from build123d import *

# Parameters (mm, degrees)
SCHIZZO1_R                   = 7
SCHIZZO1_R_2                 = 1.5
ESTRUSIONE_ESTRUSIONE1_DEPTH = 3
ESTRUSIONE_ESTRUSIONE2_DEPTH = 22
SCHIZZO3_W                   = 10
SCHIZZO3_H                   = 3
SCHIZZO3_W_2                 = 3
SCHIZZO3_H_2                 = 21.5
ESTRUSIONE_ESTRUSIONE3_DEPTH = 5


with BuildPart() as part:
    # Schizzo1 → Estrusione-Estrusione1 (new body)
    with BuildSketch(Plane.XY):
        with BuildLine():
            Line((-132.593868151, -125.596865141), (-162.593868151, -125.596865141))
            Line((-162.593868151, -125.596865141), (-162.593868151, -112.596865141))
            ThreePointArc((-162.593868151, -112.596865141), (-162.055269261, -110.529315323), (-160.576380879, -108.98732305))
            ThreePointArc((-160.576380879, -108.98732305), (-153.647502693, -93.695971479), (-165.241662126, -81.554709072))
            ThreePointArc((-165.241662126, -81.554709072), (-167.939136717, -79.887457063), (-168.993868151, -76.896865144))
            Line((-168.993868151, -76.896865144), (-168.993868151, -46.896865141))
            Line((-168.993868151, -46.896865141), (-126.193868151, -46.896865141))
            Line((-126.193868151, -46.896865141), (-126.193868151, -76.896865144))
            ThreePointArc((-126.193868151, -76.896865144), (-127.248599586, -79.887457063), (-129.946074176, -81.554709072))
            ThreePointArc((-129.946074176, -81.554709072), (-141.540233609, -93.695971479), (-134.611355423, -108.98732305))
            ThreePointArc((-134.611355423, -108.98732305), (-133.132467042, -110.529315323), (-132.593868151, -112.596865141))
            Line((-132.593868151, -112.596865141), (-132.593868151, -125.596865141))
        make_face()
        with Locations((-147.593868151, -61.896865143)):
            Circle(SCHIZZO1_R, mode=Mode.SUBTRACT)
        with Locations((-136.468868151, -68.271865143)):
            Circle(SCHIZZO1_R_2, mode=Mode.SUBTRACT)
        with Locations((-158.718868151, -68.271865143)):
            Circle(SCHIZZO1_R_2, mode=Mode.SUBTRACT)
        with Locations((-158.718868151, -55.521865143)):
            Circle(SCHIZZO1_R_2, mode=Mode.SUBTRACT)
        with Locations((-136.468868151, -55.521865143)):
            Circle(SCHIZZO1_R_2, mode=Mode.SUBTRACT)
    extrude(amount=ESTRUSIONE_ESTRUSIONE1_DEPTH)

    # Schizzo2 → Estrusione-Estrusione2 (add)
    with BuildSketch(Plane(origin=(0, 0, 0), x_dir=(-1, 0, 0), z_dir=(0, 0, -1))):
        Polygon((150.593868151, -122.596865141), (150.593868151, -121.596865141), (154.593868151, -116.196865141), (154.593868151, -115.596865141), (140.593868151, -115.596865141), (140.593868151, -116.196865141), (144.593868151, -121.596865141), (144.593868151, -122.596865141), (132.593868151, -122.596865141), (132.593868151, -125.596865141), (162.593868151, -125.596865141), (162.593868151, -122.596865141), align=None)
    extrude(amount=ESTRUSIONE_ESTRUSIONE2_DEPTH)

    # Schizzo3 → Estrusione-Estrusione3 (add)
    with BuildSketch(Plane(origin=(0, 0, 0), x_dir=(-1, 0, 0), z_dir=(0, 0, -1))):
        with Locations((147.593868151, -111.096865141)):
            Rectangle(SCHIZZO3_W, SCHIZZO3_H)
        with Locations((147.593868151, -98.846865141)):
            Rectangle(SCHIZZO3_W_2, SCHIZZO3_H_2)
    extrude(amount=ESTRUSIONE_ESTRUSIONE3_DEPTH)


solid = part.part
Design review of the part built by this model. Coordinates are the model's own, in mm. A direction names the side the tool comes from. Round coordinates to 2 decimals unless told otherwise and drop trailing zeros. Loops run counter-clockwise (first coordinate to the right, second up) from the corner with the lowest first, then second, coordinate; pieces in that order, holes last. Notation, with made-up numbers: (-3.5, -0.5) -> (33.5, -0.5) arc R34 ccw to (33.5, 33.5) -> close; hole circle Ø2 at (1, -25). An arc over 180 degrees is marked (long way). Use one line per item in the form item = value. Start each with the question number.
Q1. Wall thickness on line 1 along Z through (x, y) = (-144.5, -101.5); line 2 along Y through (x, z) = (-145, -10); line 3 along Y through (x, z) = (-152.5, 1.5): over which ranges is each line inside the solid? List them lowest first. Write a range as [from, to].
Q2. We need section A-A on z = -3.5. Give the boundary of the cut face in (x, y).
Q3. Draft analysis for pull direction Y (two halves, no side actions). For faces 1 (the face through (-142.594, -111, -2)), 2 (the face through (-148, -88.097, -2)), 3 (the face through (-157, -122.597, -11)), state which applies: +Y half, -Y half, draft (parallel to the pull), parting line (faces both ways), or undercut.
Q4. Machinability: for faces 4 (the face through (-162.594, -123, -7)), 5 (the face through (-133.15, -110.5, 1.48)), 6 (the face through (-139, -122.597, -11)), 7 (the face through (-149.094, -99, -2)), which of the approach directions +Z, -Z, +X, -X, +Y, -Y give a long, thin tool a straight path to every point of the face, cutting with its end or side? Answer none if there is none.
Q5. We need section D-D on x = -166. Give the boundary of the cut face in (y, z).
Q6. We need section B-B on z = -7.25. Give the boundary of the cut face in (x, y).
Q7. We need section C-C on y = -96.5. Give the boundary of the cut face in (x, z), then the cut area to 3 significant figures.
Q8. For pin 1 Ø1.5 at (y, z) = (-116.5, -9) entering from -X; pin 2 Ø1 at (x, z) = (-156.5, -11) entering from +Y; pin 3 Ø2.5 at (y, z) = (-100.5, -3.5) entering from +X, all flat-tipped, find the tip position at first contact; note any pin that passes through.
Calculated:
q1.line_1 = [0, 3]
q1.line_2 = [-125.6, -115.6]
q1.line_3 = [-125.6, -66.89], [-56.9, -46.9]
q2.outline = (-162.59, -125.6) -> (-132.59, -125.6) -> (-132.59, -122.6) -> (-144.59, -122.6) -> (-144.59, -121.6) -> (-140.59, -116.2) -> (-140.59, -115.6) -> (-154.59, -115.6) -> (-154.59, -116.2) -> (-150.59, -121.6) -> (-150.59, -122.6) -> (-162.59, -122.6) -> close; (-152.59, -112.6) -> (-142.59, -112.6) -> (-142.59, -109.6) -> (-146.09, -109.6) -> (-146.09, -88.1) -> (-149.09, -88.1) -> (-149.09, -109.6) -> (-152.59, -109.6) -> close
q3.face_1 = draft
q3.face_2 = +Y half
q3.face_3 = undercut
q4.face_4 = +Z, -Z, -X, -Y
q4.face_5 = +Z, -Z, +X
q4.face_6 = -Z, +X
q4.face_7 = -Z, -X, +Y
q5.outline = (-81.32, 0) -> (-46.9, 0) -> (-46.9, 3) -> (-81.32, 3) -> close
q6.outline = (-162.59, -125.6) -> (-132.59, -125.6) -> (-132.59, -122.6) -> (-144.59, -122.6) -> (-144.59, -121.6) -> (-140.59, -116.2) -> (-140.59, -115.6) -> (-154.59, -115.6) -> (-154.59, -116.2) -> (-150.59, -121.6) -> (-150.59, -122.6) -> (-162.59, -122.6) -> close
q7.outline = (-153.44, 0) -> (-149.09, 0) -> (-149.09, -5) -> (-146.09, -5) -> (-146.09, 0) -> (-141.75, 0) -> (-141.75, 3) -> (-153.44, 3) -> close
q7.area = 50.1 mm²
q8.pin_1 = -154.59
q8.pin_2 = -122.6
q8.pin_3 = -146.09
